```python
from build123d import *

# Parameters (mm, degrees)
SKETCH_1_W          = 80
SKETCH_1_H          = 34
EXTRUDE_1_DEPTH     = 4
CUT_EXTRUDE_1_REACH = 45.646
SKETCH_2_R          = 1.6
SKETCH_3_W          = 40
SKETCH_3_H          = 24
EXTRUDE_2_DEPTH     = 4
SKETCH_4_W          = 20
SKETCH_4_H          = 6
EXTRUDE_3_DEPTH     = 15
SKETCH_5_W          = 40
SKETCH_5_H          = 23.790626796
EXTRUDE_4_DEPTH     = 3
CUT_EXTRUDE_2_REACH = 74.883
SKETCH_6_R          = 2.1


with BuildPart() as part:
    # 草图1 → 凸台-拉伸1 (new body)
    with BuildSketch(Plane(origin=(0, 0, 0), x_dir=(1, 0, 0), z_dir=(0, 1, 0))):
        Rectangle(SKETCH_1_W, SKETCH_1_H)
    extrude(amount=EXTRUDE_1_DEPTH)

    # 草图2 → 切除-拉伸1 (cut, up to next)
    with BuildSketch(Plane(origin=(0, 4, 0), x_dir=(1, 0, 0), z_dir=(0, 1, 0)), mode=Mode.PRIVATE) as cut_extrude_1_sk1:
        with Locations(Location((-22.5, 7, 0), (0, 0, 270))):
            Circle(SKETCH_2_R)
    cut_extrude_1_tool1 = extrude(cut_extrude_1_sk1.sketch, amount=-CUT_EXTRUDE_1_REACH, mode=Mode.PRIVATE) & part.part
    # 草图2 → 切除-拉伸1 (cut, up to next)
    with BuildSketch(Plane(origin=(0, 4, 0), x_dir=(1, 0, 0), z_dir=(0, 1, 0)), mode=Mode.PRIVATE) as cut_extrude_1_sk2:
        with Locations(Location((22.5, 7, 0), (0, 0, 270))):
            Circle(SKETCH_2_R)
    cut_extrude_1_tool2 = extrude(cut_extrude_1_sk2.sketch, amount=-CUT_EXTRUDE_1_REACH, mode=Mode.PRIVATE) & part.part
    add(cut_extrude_1_tool1.solids().sort_by_distance((-22.5, 4, -7))[0], mode=Mode.SUBTRACT)
    add(cut_extrude_1_tool2.solids().sort_by_distance((22.5, 4, -7))[0], mode=Mode.SUBTRACT)

    # 草图3 → 凸台-拉伸2 (add)
    with BuildSketch(Plane.XY.offset(17)):
        with Locations((0, 12)):
            Rectangle(SKETCH_3_W, SKETCH_3_H)
    extrude(amount=EXTRUDE_2_DEPTH)

    # 草图4 → 凸台-拉伸3 (add)
    with BuildSketch(Plane.XY.offset(21)):
        with Locations((-0.061987537, 3)):
            Rectangle(SKETCH_4_W, SKETCH_4_H)
    extrude(amount=EXTRUDE_3_DEPTH)

    # 草图5 → 凸台-拉伸4 (add)
    with BuildSketch(Plane.XY.offset(36)):
        with Locations((0, 11.895313398)):
            Rectangle(SKETCH_5_W, SKETCH_5_H)
    extrude(amount=EXTRUDE_4_DEPTH)

    # 切除-拉伸2: up to this face of the body (flat: up to its plane)
    cut_extrude_2_end = Plane(part.part.faces().sort_by_distance((0, 14, 17))[0])
    # 草图6 → 切除-拉伸2 (cut, up to the picked face)
    with BuildSketch(Plane.XY.offset(39), mode=Mode.PRIVATE) as cut_extrude_2_sk1:
        with Locations((-13.5, 11.895313398)):
            Circle(SKETCH_6_R)
    cut_extrude_2_tool1 = split(extrude(cut_extrude_2_sk1.sketch, amount=-CUT_EXTRUDE_2_REACH, mode=Mode.PRIVATE), bisect_by=cut_extrude_2_end, keep=Keep.BOTH, mode=Mode.PRIVATE)
    # 草图6 → 切除-拉伸2 (cut, up to the picked face)
    with BuildSketch(Plane.XY.offset(39), mode=Mode.PRIVATE) as cut_extrude_2_sk2:
        with Locations((-5.5, 11.895313398)):
            Circle(SKETCH_6_R)
    cut_extrude_2_tool2 = split(extrude(cut_extrude_2_sk2.sketch, amount=-CUT_EXTRUDE_2_REACH, mode=Mode.PRIVATE), bisect_by=cut_extrude_2_end, keep=Keep.BOTH, mode=Mode.PRIVATE)
    # 草图6 → 切除-拉伸2 (cut, up to the picked face)
    with BuildSketch(Plane.XY.offset(39), mode=Mode.PRIVATE) as cut_extrude_2_sk3:
        with Locations((5.5, 11.895313398)):
            Circle(SKETCH_6_R)
    cut_extrude_2_tool3 = split(extrude(cut_extrude_2_sk3.sketch, amount=-CUT_EXTRUDE_2_REACH, mode=Mode.PRIVATE), bisect_by=cut_extrude_2_end, keep=Keep.BOTH, mode=Mode.PRIVATE)
    # 草图6 → 切除-拉伸2 (cut, up to the picked face)
    with BuildSketch(Plane.XY.offset(39), mode=Mode.PRIVATE) as cut_extrude_2_sk4:
        with Locations((13.5, 11.895313398)):
            Circle(SKETCH_6_R)
    cut_extrude_2_tool4 = split(extrude(cut_extrude_2_sk4.sketch, amount=-CUT_EXTRUDE_2_REACH, mode=Mode.PRIVATE), bisect_by=cut_extrude_2_end, keep=Keep.BOTH, mode=Mode.PRIVATE)
    add(cut_extrude_2_tool1.solids().sort_by(Axis((-13.5, 11.895313, 39), (0, 0, -1)))[0], mode=Mode.SUBTRACT)
    add(cut_extrude_2_tool2.solids().sort_by(Axis((-5.5, 11.895313, 39), (0, 0, -1)))[0], mode=Mode.SUBTRACT)
    add(cut_extrude_2_tool3.solids().sort_by(Axis((5.5, 11.895313, 39), (0, 0, -1)))[0], mode=Mode.SUBTRACT)
    add(cut_extrude_2_tool4.solids().sort_by(Axis((13.5, 11.895313, 39), (0, 0, -1)))[0], mode=Mode.SUBTRACT)


solid = part.part
```
Work out the finished part from the listing and answer in its coordinate system (mm). A direction names the side the tool comes from. Coordinates: 2 decimals unless noted, no trailing zeros. Loops run counter-clockwise (first coordinate to the right, second up) from the corner with the lowest first, then second, coordinate; pieces in that order, holes last.
1) For faces 1 (the flat face through (20, 12, 19)), 2 (the flat face through (-30, 2, 17)), 3 (the cylindrical face through (-20.914, 2.028, -7.208)), 4 (the flat face through (9.938, 3, 28)), determine the directions among +Z, -Z, +X, -X, +Y, -Y from which every point of the face is accessible in a straight line to the end or side of a thin tool.
Results:
face 1: +Z, +X, +Y, -Y
face 2: +Z, -X, +Y, -Y
face 3: +Y, -Y
face 4: +X, +Y, -Y
2) Section D-D (x = -5.5) is taken. Give the vertices of the cut face in (y, z), plus the area to 3 significant figures.
Results:
outline: (0, -17) - (4, -17) - (4, 17) - (9.8, 17) - (9.8, 21) - (6, 21) - (6, 36) - (9.8, 36) - (9.8, 39) - (0, 39) - close; (14, 17) - (24, 17) - (24, 21) - (14, 21) - close; (14, 36) - (23.79, 36) - (23.79, 39) - (14, 39) - close
area: 364 mm2
3) Flat-ended cylindrical pins translate along their axes: pin 1 (2.5 mm diameter, centred on x = -22.5, z = -7, fed in from +Y); pin 2 (4 mm diameter, centred on x = -7.5, z = 22.5, fed in from +Y); pin 3 (4 mm diameter, centred on x = 22.5, z = 14, fed in from +Y); pin 4 (2.5 mm diameter, centred on y = 12.5, z = 37.5, fed in from +X). Find the tip coordinate at first contact, or state that the pin passes through.
Results:
pin 1: passes through
pin 2: stops at y = 24
pin 3: stops at y = 4
pin 4: stops at x = 20
4) Section C-C (y = 15.5) is taken. Give the vertices of the cut face in (x, z), plus the area to 3 significant figures.
Results:
outline: (-20, 17) - (20, 17) - (20, 21) - (-20, 21) - close; (-20, 36) - (20, 36) - (20, 39) - (-20, 39) - close
area: 280 mm2
5) Section A-A (x = -22.5) is taken. Give the vertices of the cut face in (y, z), plus the area to 3 significant figures.
Results:
outline: (0, -17) - (4, -17) - (4, -8.6) - (0, -8.6) - close; (0, -5.4) - (4, -5.4) - (4, 17) - (0, 17) - close
area: 123 mm2
6) Consider probe 1 along X at (y, z) = (2.3, -7); probe 2 along Y at (x, z) = (-5.5, 19.5); probe 3 along Z at (x, y) = (-3, 18.25). Determine where each line is inside the solid, lowest interval first.
Results:
probe 1: x = -40 to -24.1, -20.9 to 20.9, 24.1 to 40
probe 2: y = 0 to 9.8, 14 to 24
probe 3: z = 17 to 21, 36 to 39
7) For a pull along X with two mould halves and no side action, classify faces 5 (the flat face through (-10.062, 3, 28)), 6 (the cylindrical face through (24.086, 2.028, -7.208)), 7 (the flat face through (30, 2, 17)) as +X half, -X half, draft (parallel to the pull), parting line (faces both ways), or undercut.
Results:
face 5: -X half
face 6: undercut
face 7: draft
8) Section B-B (z = -7) is taken. Give the vertices of the cut face in (x, y).
Results:
outline: (-40, 0) - (-24.1, 0) - (-24.1, 4) - (-40, 4) - close; (-20.9, 0) - (20.9, 0) - (20.9, 4) - (-20.9, 4) - close; (24.1, 0) - (40, 0) - (40, 4) - (24.1, 4) - close
